```python
from build123d import *

# Parameters (mm, degrees)
BOSS_EXTRU_2_DEPTH = 5
CHANFREIN1_SIZE    = 0.5


with BuildPart() as part:
    # Esquisse1 → Boss.-Extru.2 (new body)
    with BuildSketch(Plane.XY):
        with BuildLine():
            Line((0, 24), (0, 27.5))
            ThreePointArc((0, 27.5), (-27.5, 0), (0, -27.5))
            Line((0, -27.5), (0, -24))
            ThreePointArc((0, -24), (-1.078192933, -23.542832681), (-1.499166435, -22.45))
            ThreePointArc((-1.499166435, -22.45), (-15.909902577, -15.909902577), (-22.45, -1.499166435))
            ThreePointArc((-22.45, -1.499166435), (-24, 0), (-22.45, 1.499166435))
            ThreePointArc((-22.45, 1.499166435), (-15.909902577, 15.909902577), (-1.499166435, 22.45))
            ThreePointArc((-1.499166435, 22.45), (-1.078192933, 23.542832681), (0, 24))
        make_face()
        with BuildLine():
            ThreePointArc((0, 21), (-1.042832681, 21.421807067), (-1.499166435, 22.45))
            ThreePointArc((-1.499166435, 22.45), (-15.909902577, 15.909902577), (-22.45, 1.499166435))
            ThreePointArc((-22.45, 1.499166435), (-21.421807067, 1.042832681), (-21, 0))
            ThreePointArc((-21, 0), (-21.421807067, -1.042832681), (-22.45, -1.499166435))
            ThreePointArc((-22.45, -1.499166435), (-15.909902577, -15.909902577), (-1.499166435, -22.45))
            ThreePointArc((-1.499166435, -22.45), (-1.042832681, -21.421807067), (0, -21))
            Line((0, -21), (0, -2.51))
            ThreePointArc((0, -2.51), (-2.51, 0), (0, 2.51))
            Line((0, 2.51), (0, 21))
        make_face()
        with BuildLine():
            ThreePointArc((1.499166435, 22.45), (1.042832681, 21.421807067), (0, 21))
            Line((0, 21), (0, 2.51))
            ThreePointArc((0, 2.51), (1.774838021, 1.774838021), (2.51, 0))
            ThreePointArc((2.51, 0), (1.774838021, -1.774838021), (0, -2.51))
            Line((0, -2.51), (0, -21))
            ThreePointArc((0, -21), (1.042832681, -21.421807067), (1.499166435, -22.45))
            ThreePointArc((1.499166435, -22.45), (15.909902577, -15.909902577), (22.45, -1.499166435))
            ThreePointArc((22.45, -1.499166435), (21, 0), (22.45, 1.499166435))
            ThreePointArc((22.45, 1.499166435), (15.909902577, 15.909902577), (1.499166435, 22.45))
        make_face()
        with BuildLine():
            ThreePointArc((27.5, 0), (19.445436483, 19.445436483), (0, 27.5))
            Line((0, 27.5), (0, 24))
            ThreePointArc((0, 24), (1.060660172, 23.560660172), (1.5, 22.5))
            ThreePointArc((1.5, 22.5), (1.499791594, 22.474996526), (1.499166435, 22.45))
            ThreePointArc((1.499166435, 22.45), (15.909902577, 15.909902577), (22.45, 1.499166435))
            ThreePointArc((22.45, 1.499166435), (23.542832681, 1.078192933), (24, 0))
            ThreePointArc((24, 0), (23.542832681, -1.078192933), (22.45, -1.499166435))
            ThreePointArc((22.45, -1.499166435), (15.909902577, -15.909902577), (1.499166435, -22.45))
            ThreePointArc((1.499166435, -22.45), (1.499791594, -22.474996526), (1.5, -22.5))
            ThreePointArc((1.5, -22.5), (1.060660172, -23.560660172), (0, -24))
            Line((0, -24), (0, -27.5))
            ThreePointArc((0, -27.5), (19.445436483, -19.445436483), (27.5, 0))
        make_face()
    extrude(amount=BOSS_EXTRU_2_DEPTH)

    # Cong_1: read off the stored shape, not the designer's step
    # Cong_1 outline → Cong_1 (revolve, cut)
    with BuildSketch(Plane.XZ):
        with BuildLine():
            ThreePointArc((26.5, 5), (27.207106781, 4.707106781), (27.5, 4))
            Line((27.5, 4), (27.5, 5))
            Line((27.5, 5), (26.5, 5))
        make_face()
        with BuildLine():
            Line((27.5, 0), (27.5, 1))
            ThreePointArc((27.5, 1), (27.207106781, 0.292893219), (26.5, 0))
            Line((26.5, 0), (27.5, 0))
        make_face()
    revolve(axis=Axis((0, 0, 0), (0, 0, 1)), mode=Mode.SUBTRACT)

    # Chanfrein1
    chanfrein1_edges = [part.edges().sort_by_distance(p)[0] for p in [
        (0, 21, 5),
        (22.55, 1.499166435, 5),
        (-1.499166435, -22.55, 5),
        (-22.55, -1.499166435, 5),
    ]]
    chamfer(chanfrein1_edges, length=CHANFREIN1_SIZE)


solid = part.part
```
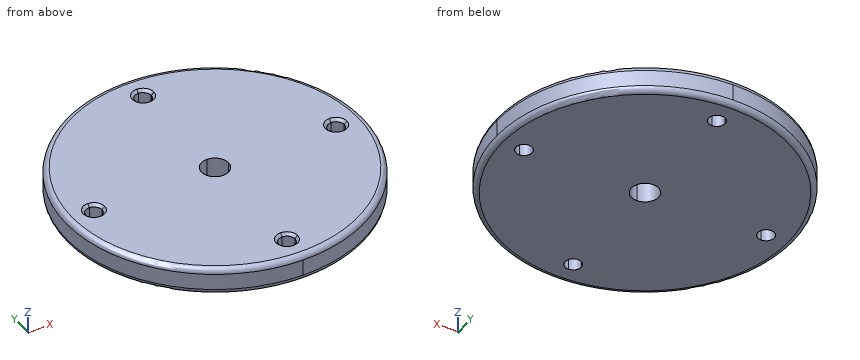
The model under review builds one solid part; all positions refer to its coordinate system, in mm. Give positions to 0.01 mm unless a question says otherwise; leave off trailing zeros. Write each loop counter-clockwise with the first axis right and the second up, starting at its lowest first coordinate (ties: lowest second). Pieces come first, ordered by that corner, then holes.
(1) To check wall thickness, follow L1, parallel to Y at x = 1, z = 1.05; L2, parallel to Y at x = -21.5, z = 0.6; L3, parallel to Z at x = -20, y = -17.5. State the ranges of each line that lie inside material, in increasing order.
(2) Consider section A-A, the plane z = 2.9. Give the boundary of the cut face in (x, y), and give its area (3 significant figures).
(3) For P1, Ø1, axis at y = 17, z = 1, coming from the -X side; P2, Ø1.5, axis at x = 20, z = 1, coming from the +Y side; P3, Ø1, axis at y = 2.5, z = 4.5, coming from the -X side, all flat-tipped, find the tip position at first contact; note any pin that passes through.
Returned:
1. L1: y = -27.48 to -23.62, -21.38 to -2.3, 2.3 to 21.38, 23.62 to 27.48
1. L2: y = -17.01 to -1.12, 1.12 to 17.01
1. L3: z = 0 to 5
2. outline: circle Ø55 at (0, 0); hole circle Ø3 at (-22.5, 0); hole circle Ø5.02 at (0, 0); hole (1.5, -22.5) arc R1.5 ccw to (1.5, -22.45) arc R1.5 ccw (long way) to start; hole (1.5, 22.45) arc R1.5 ccw to (1.5, 22.5) arc R1.5 ccw (long way) to start; hole circle Ø3 at (22.5, 0)
2. area: 2,330 mm2
3. P1: stops at x = -22
3. P2: stops at y = 19.64
3. P3: stops at x = -27.41
